```python
from build123d import *

# Parameters (mm, degrees)
IZIM1_R                     = 10
Y_KSEKLIK_EKSTR_ZYON2_DEPTH = 70
IZIM4_R                     = 2.9
KES_EKSTR_ZYON1_DEPTH       = 10
IZIM6_R                     = 2.9
KES_EKSTR_ZYON2_DEPTH       = 10


with BuildPart() as part:
    # Çizim1 → Yükseklik-Ekstrüzyon2 (new body)
    with BuildSketch(Plane.XY):
        Polygon((34.558000078, -9.253153646), (0.014602542, -15.067885605), (-34.611999922, -9.444150005), (-34.611999922, 19.740712429), (34.558000078, 19.740712429), align=None)
        with Locations((-24.214579028, 6.217247179)):
            Circle(IZIM1_R, mode=Mode.SUBTRACT)
        Circle(IZIM1_R, mode=Mode.SUBTRACT)
        with Locations((24.214579028, 6.217247179)):
            Circle(IZIM1_R, mode=Mode.SUBTRACT)
    extrude(amount=Y_KSEKLIK_EKSTR_ZYON2_DEPTH)

    # Çizim4 → Kes-Ekstrüzyon1 (cut, along a direction that is not the sketch's normal)
    with BuildSketch(Plane(origin=(-2.383921421, -14.678339313, 0), x_dir=(0.9870666640552537, -0.1603103262763605, 0), z_dir=(-0.1603103262763605, -0.9870666640552537, 0))):
        with Locations((-10.65035653, 60)):
            Circle(IZIM4_R)
        with Locations((-10.65035653, 10)):
            Circle(IZIM4_R)
    extrude(amount=-KES_EKSTR_ZYON1_DEPTH, dir=(0, -1, 0), mode=Mode.SUBTRACT)

    # Çizim6 → Kes-Ekstrüzyon2 (cut, along a direction that is not the sketch's normal)
    with BuildSketch(Plane(origin=(2.466908381, -14.655085992, 0), x_dir=(0.9861264495259806, 0.16599586002453082, 0), z_dir=(0.16599586002453082, -0.9861264495259807, 0))):
        with Locations((10.542572723, 60)):
            Circle(IZIM6_R)
        with Locations((10.542572723, 10)):
            Circle(IZIM6_R)
    extrude(amount=-KES_EKSTR_ZYON2_DEPTH, dir=(0, -1, 0), mode=Mode.SUBTRACT)


solid = part.part
```
The listing builds one solid part. Answer for the finished solid, in the listing's coordinates (mm). Coordinates: 2 decimals unless noted, no trailing zeros. Loops run counter-clockwise (first coordinate to the right, second up) from the corner with the lowest first, then second, coordinate; pieces in that order, holes last. Notation, with made-up numbers: (60, 12) - (64, 12) arc R24 cw to (64, 36) - close; hole circle Ø4 at (58.25, 48). An arc over 180 degrees is marked (long way). Use a Markdown table: item, result. Add a question column.
1) The part is cut by section B-B, the plane y = 0. Give the vertices of the cut face in (x, z), and give its area (3 significant figures).
2) The part is cut by section C-C, the plane z = 23.5. Give the vertices of the cut face in (x, y).
3) Given pin 1 (3 mm diameter, centred on x = -16, y = 5, fed in from +Z); pin 2 (1.5 mm diameter, centred on x = 24.5, z = 43.5, fed in from -Y), each flat-ended and moving along its own axis, determine where each tip first touches the part or whether it passes through.
4) The mould has two halves that part along Y. Classify faces 1 (the cylindrical face through (-32.15, 0.13, 34.51)), 2 (the cylindrical face through (-2.17, -9.76, 34.51)), 3 (the flat face through (0.5, 10.3, 70)), 4 (the flat face through (-17.056, -12.295, 34.51)): released by +Y, released by -Y, zero draft, split by the parting line, or undercut.
5) The part is cut by section D-D, the plane x = 23.5. Give the vertices of the cut face in (y, z).
6) Find the intervals of material crossed by line 1 (Y direction, x = 0, z = 44); line 2 (X direction, y = 15.5, z = 41); line 3 (X direction, y = 3, z = 37), in increasing order.
7) The part is cut by section A-A, the plane x = -22. Give the vertices of the cut face in (y, z).
Here are the results:
| question | item | result |
|---|---|---|
| 1 | outline | (-34.61, 0) - (-32.05, 0) - (-32.05, 70) - (-34.61, 70) - close; (-16.38, 0) - (-10, 0) - (-10, 70) - (-16.38, 70) - close; (10, 0) - (16.38, 0) - (16.38, 70) - (10, 70) - close; (32.05, 0) - (34.56, 0) - (34.56, 70) - (32.05, 70) - close |
| 1 | area | 1,250 mm^2 |
| 2 | outline | (-34.61, -9.44) - (0.01, -15.07) - (34.56, -9.25) - (34.56, 19.74) - (-34.61, 19.74) - close; hole circle Ø20 at (-24.21, 6.22); hole circle Ø20 at (0, 0); hole circle Ø20 at (24.21, 6.22) |
| 3 | pin 1 | passes through |
| 3 | pin 2 | stops at y = -11.07 |
| 4 | face 1 | undercut |
| 4 | face 2 | undercut |
| 4 | face 3 | zero draft |
| 4 | face 4 | released by -Y |
| 5 | outline | (-11.11, 0) - (-3.76, 0) - (-3.76, 70) - (-11.11, 70) - close; (16.19, 0) - (19.74, 0) - (19.74, 70) - (16.19, 70) - close |
| 6 | line 1 | y = -15.07 to -10, 10 to 19.74 |
| 6 | line 2 | x = -34.61 to -27.93, -20.5 to 20.5, 27.93 to 34.56 |
| 6 | line 3 | x = -34.61 to -33.68, -14.75 to -9.54, 9.54 to 14.75, 33.68 to 34.56 |
| 7 | outline | (-11.49, 0) - (-3.53, 0) - (-3.53, 70) - (-11.49, 70) - close; (15.97, 0) - (19.74, 0) - (19.74, 70) - (15.97, 70) - close |
